from build123d import *

# Parameters (mm, degrees)
SKETCH_R   = 4
SKETCH_R_2 = 1.6
SKETCH_R_3 = 25
PAD_DEPTH  = 3
FILLET_R   = 10


with BuildPart() as part:
    # Sketch → Pad (new body)
    with BuildSketch(Plane.XY):
        with BuildLine():
            ThreePointArc((0, 12), (-12, 0), (0, -12))
            Line((0, -12), (18.5, -32))
            Line((77.5, -32), (18.5, -32))
            Line((96, -12), (77.5, -32))
            ThreePointArc((96, -12), (108, 0), (96, 12))
            Line((77.5, 29.5), (96, 12))
            Line((18.5, 29.5), (77.5, 29.5))
            Line((18.5, 29.5), (0, 12))
        make_face()
        Circle(SKETCH_R, mode=Mode.SUBTRACT)
        with Locations((96, 0)):
            Circle(SKETCH_R, mode=Mode.SUBTRACT)
        with Locations((25.5, -25)):
            Circle(SKETCH_R_2, mode=Mode.SUBTRACT)
        with Locations((70.5, -25)):
            Circle(SKETCH_R_2, mode=Mode.SUBTRACT)
        with Locations((25.5, 22.5)):
            Circle(SKETCH_R_2, mode=Mode.SUBTRACT)
        with Locations((70.5, 22.5)):
            Circle(SKETCH_R_2, mode=Mode.SUBTRACT)
        with Locations((48, -1.25)):
            Circle(SKETCH_R_3, mode=Mode.SUBTRACT)
    extrude(amount=PAD_DEPTH)

    # Fillet
    fillet_edges = [part.edges().sort_by_distance(p)[0] for p in [
        (77.5, -32, 1.5),
        (18.5, -32, 1.5),
        (77.5, 29.5, 1.5),
        (18.5, 29.5, 1.5),
    ]]
    fillet(fillet_edges, radius=FILLET_R)


solid = part.part
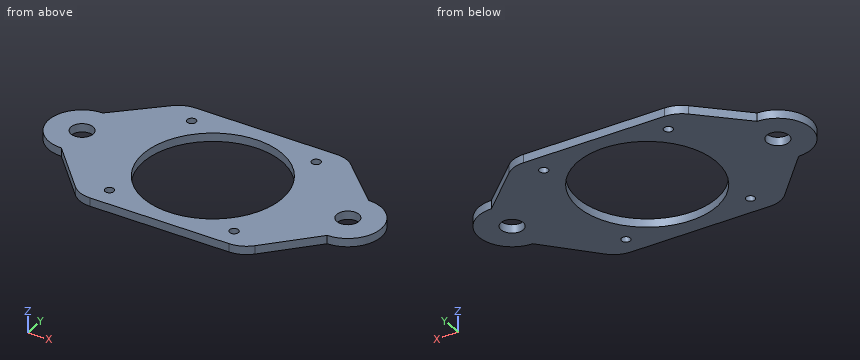
The listing builds one solid part. Answer for the finished solid, in the listing's coordinates (mm). Give positions to 0.01 mm unless a question says otherwise; leave off trailing zeros. Write each loop counter-clockwise with the first axis right and the second up, starting at its lowest first coordinate (ties: lowest second). Pieces come first, ordered by that corner, then holes.
Item 1: Section D-D, the plane x = 70.5 is taken. Write down the section's boundary in (y, z), plus the area to 3 significant figures.
Item 2: Find the intervals of material crossed by line 1 along Y through (x, z) = (96, 1.2); line 2 along Y through (x, z) = (25.5, 1.7); line 3 along X through (y, z) = (5, 2.8), in increasing order.
Item 3: Section B-B, the plane z = 0.45 is taken. Write down the section's boundary in (x, y), plus the area to 3 significant figures.
Item 4: Section A-A, the plane x = 48 is taken. Write down the section's boundary in (y, z), plus the area to 3 significant figures.
Item 5: A flat-ended cylindrical pin translates along its axis: P1, Ø7, axis at x = 96, y = 0, coming from the +Z side. Find the tip coordinate at first contact, or state that the pin passes through.
Item 6: Section C-C, the plane y = -25 is taken. Write down the section's boundary in (x, z) (3 decimals), plus the area to 3 significant figures.
Completed:
1. outline: (-32, 0) - (-26.6, 0) - (-26.6, 3) - (-32, 3) - close; (-23.4, 0) - (-12.15, 0) - (-12.15, 3) - (-23.4, 3) - close; (9.65, 0) - (20.9, 0) - (20.9, 3) - (9.65, 3) - close; (24.1, 0) - (29.5, 0) - (29.5, 3) - (24.1, 3) - close
1. area: 99.9 mm2
2. line 1: y = -12 to -4, 4 to 12
2. line 2: y = -32 to -26.6, -23.4 to -12.15, 9.65 to 20.9, 24.1 to 29.5
2. line 3: x = -10.91 to 23.79, 72.21 to 106.91
3. outline: (0, -12) - (15.53, -28.79) arc R10 ccw to (22.87, -32) - (73.13, -32) arc R10 ccw to (80.47, -28.79) - (96, -12) arc R12 ccw to (96, 12) - (80.39, 26.76) arc R10 ccw to (73.52, 29.5) - (22.48, 29.5) arc R10 ccw to (15.61, 26.76) - (0, 12) arc R12 ccw to start; hole circle Ø8 at (0, 0); hole circle Ø50 at (48, -1.25); hole circle Ø3.2 at (25.5, -25); hole circle Ø3.2 at (25.5, 22.5); hole circle Ø3.2 at (70.5, -25); hole circle Ø3.2 at (70.5, 22.5); hole circle Ø8 at (96, 0)
3. area: 3,560 mm2
4. outline: (-32, 0) - (-26.25, 0) - (-26.25, 3) - (-32, 3) - close; (23.75, 0) - (29.5, 0) - (29.5, 3) - (23.75, 3) - close
4. area: 34.5 mm2
5. P1: passes through
6. outline: (12.025, 0) - (23.9, 0) - (23.9, 3) - (12.025, 3) - close; (27.1, 0) - (40.194, 0) - (40.194, 3) - (27.1, 3) - close; (55.806, 0) - (68.9, 0) - (68.9, 3) - (55.806, 3) - close; (72.1, 0) - (83.975, 0) - (83.975, 3) - (72.1, 3) - close
6. area: 150 mm2
